```python
from build123d import *

# Parameters (mm, degrees)
SALIENTE_EXTRUIR1_DEPTH = 3
CROQUIS_BARRIDOS_R      = 1.45
CROQUIS_BARRIDOS_R_2    = 5.5
CROQUIS_BARRIDOS_R_3    = 4.5
CROQUIS_BARRIDOS_R_4    = 1.5
CORTAR_EXTRUIR1_DEPTH   = 3
REDONDEO1_R             = 3
REDONDEO2_R             = 1


with BuildPart() as part:
    # Croquis base → Saliente-Extruir1 (new body)
    with BuildSketch(Plane(origin=(0, 0, 0), x_dir=(1, 0, 0), z_dir=(0, 1, 0))):
        Polygon((-27.25, 11), (-19.65, 11), (-9.65, 21), (4.35, 21), (14.35, 11), (27.25, 11), (27.25, -11), (14.35, -11), (4.85, -24.8), (-10.15, -24.8), (-19.65, -11), (-27.25, -11), align=None)
    extrude(amount=SALIENTE_EXTRUIR1_DEPTH)

    # Croquis barridos → Cortar-Extruir1 (cut)
    with BuildSketch(Plane(origin=(0, 3, 0), x_dir=(1, 0, 0), z_dir=(0, 1, 0))):
        with Locations(Location((-14.88, -0.25, 0), (0, 0, 270))):
            Circle(CROQUIS_BARRIDOS_R)
        with Locations(Location((-1, 0, 0), (0, 0, 270))):
            Circle(CROQUIS_BARRIDOS_R_2)
        with Locations(Location((10, 0, 0), (0, 0, 270))):
            Circle(CROQUIS_BARRIDOS_R_3)
        with Locations(Location((-24.25, 5, 0), (0, 0, 270))):
            Circle(CROQUIS_BARRIDOS_R_4)
        with Locations(Location((24.25, 5, 0), (0, 0, 90))):
            Circle(CROQUIS_BARRIDOS_R_4)
        with Locations(Location((24.25, -5, 0), (0, 0, 270))):
            Circle(CROQUIS_BARRIDOS_R_4)
        with Locations(Location((-24.25, -5, 0), (0, 0, 90))):
            Circle(CROQUIS_BARRIDOS_R_4)
        with Locations(Location((-8.65, -17.8, 0), (0, 0, 270))):
            Circle(CROQUIS_BARRIDOS_R_4)
        with Locations(Location((-7.15, 18, 0), (0, 0, 270))):
            Circle(CROQUIS_BARRIDOS_R)
        with Locations(Location((3.35, -17.8, 0), (0, 0, 90))):
            Circle(CROQUIS_BARRIDOS_R_4)
        with Locations(Location((1.85, 18, 0), (0, 0, 90))):
            Circle(CROQUIS_BARRIDOS_R)
        with BuildLine():
            Line((-4.15, -24.8), (-1.15, -24.8))
            ThreePointArc((-1.15, -24.8), (-2.65, -23.877), (-4.15, -24.8))
        make_face()
    extrude(amount=-CORTAR_EXTRUIR1_DEPTH, mode=Mode.SUBTRACT)

    # Redondeo1
    redondeo1_edges = [part.edges().sort_by_distance(p)[0] for p in [
        (4.85, 1.5, 24.8),
        (-10.15, 1.5, 24.8),
        (-27.25, 1.5, 11),
        (-27.25, 1.5, -11),
        (-9.65, 1.5, -21),
        (4.35, 1.5, -21),
        (27.25, 1.5, -11),
        (27.25, 1.5, 11),
    ]]
    fillet(redondeo1_edges, radius=REDONDEO1_R)

    # Redondeo2
    redondeo2_edges = [part.edges().sort_by_distance(p)[0] for p in [
        (-4.15, 1.5, 24.8),
        (-1.15, 1.5, 24.8),
    ]]
    fillet(redondeo2_edges, radius=REDONDEO2_R)


solid = part.part
```
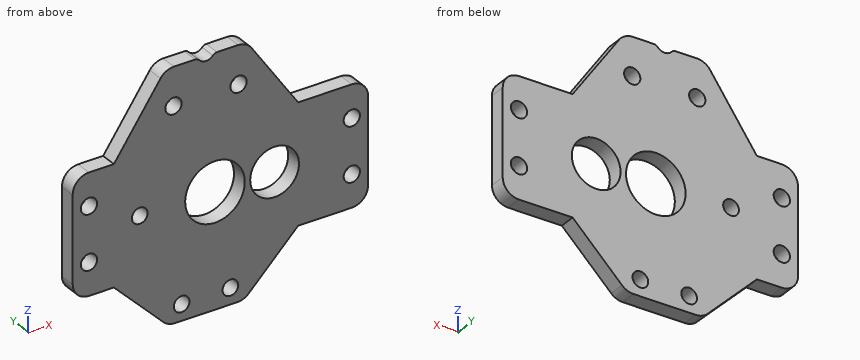
Read the model definition and answer for the solid it produces. Units are mm, in the model's axes. Give positions to 0.01 mm unless a question says otherwise; leave off trailing zeros. Write each loop counter-clockwise with the first axis right and the second up, starting at its lowest first coordinate (ties: lowest second). Pieces come first, ordered by that corner, then holes. Notation, with made-up numbers: (21.5, 43) -> (41.5, 43) arc R16 ccw to (41.5, 59) -> close; hole circle Ø6 at (4.5, 10.5). An arc over 180 degrees is marked (long way). Answer as a JSON object with one key per item and string values.
1) Section C-C on z = 17 is taken. Write down the section's boundary in (x, y).
Findings below:
{"outline": "(-15.52, 0) -> (-9.92, 0) -> (-9.92, 3) -> (-15.52, 3) -> close; (-7.38, 0) -> (2.08, 0) -> (2.08, 3) -> (-7.38, 3) -> close; (4.62, 0) -> (10.22, 0) -> (10.22, 3) -> (4.62, 3) -> close"}
2) A flat-ended cylindrical pin translates along its axis: pin 1 Ø0.9 at (x, y) = (-23, 1) entering from +Z. Find the tip coordinate at first contact, or state that the pin passes through.
Findings below:
{"pin 1": "stops at z = 11"}
3) Section B-B on x = 10 is taken. Write down the section's boundary in (y, z).
Findings below:
{"outline": "(0, -15.35) -> (3, -15.35) -> (3, -4.5) -> (0, -4.5) -> close; (0, 4.5) -> (3, 4.5) -> (3, 17.32) -> (0, 17.32) -> close"}
4) Section D-D on y = 1.7 is taken. Count the separate pieces of the cut face and the enclosed holes in it, then the cut area to 3 significant figures.
Findings below:
{"separate pieces": "1", "enclosed holes": "11", "area": "1,550 mm^2"}
5) Straight lines are drawn through the part: probe 1 along X at (y, z) = (0.5, 1.5); probe 2 along Z at (x, y) = (-7.5, 0.75); probe 3 along X at (y, z) = (2.7, 5). For each, find the intervals that lie inside material, in ascending order. Write a range as from..to.
Findings below:
{"probe 1": "x = -27.25..-15.61, -14.15..-6.29, 4.29..5.76, 14.24..27.25", "probe 2": "z = -21..-19.41, -16.59..16.84, 18.76..24.8", "probe 3": "x = -27.25..-25.75, -22.75..-3.29, 1.29..22.75, 25.75..27.25"}
6) Section A-A on z = 0 is taken. Write down the section's boundary in (x, y), then the cut area to 3 significant figures.
Findings below:
{"outline": "(-27.25, 0) -> (-16.31, 0) -> (-16.31, 3) -> (-27.25, 3) -> close; (-13.45, 0) -> (-6.5, 0) -> (-6.5, 3) -> (-13.45, 3) -> close; (4.5, 0) -> (5.5, 0) -> (5.5, 3) -> (4.5, 3) -> close; (14.5, 0) -> (27.25, 0) -> (27.25, 3) -> (14.5, 3) -> close", "area": "94.9 mm^2"}
